```python
from build123d import *

# Parameters (mm, degrees)
F0_W     = 208
F0_H     = 115
F0_W_2   = 197.84
F0_H_2   = 109.92
F1_DEPTH = 4
F2_R     = 6
F3_SIZE  = 12.7
F4_W     = 15
F4_H     = 4
F5_DEPTH = 6
F6_W     = 15
F6_H     = 4
F7_DEPTH = 6
F8_R     = 3


with BuildPart() as f1:
    # F0 (on Top) → F1 (new body)
    with BuildSketch(Plane.XY):
        with Locations((104, 57.5)):
            Rectangle(F0_W, F0_H)
        with Locations((104, 57.5)):
            Rectangle(F0_W_2, F0_H_2, mode=Mode.SUBTRACT)
    extrude(amount=F1_DEPTH)

    # F2
    f2_edges = [f1.edges().sort_by_distance(p)[0] for p in [
        (0, 115, 2),
        (208, 115, 2),
        (208, 0, 2),
        (0, 0, 2),
    ]]
    fillet(f2_edges, radius=F2_R)

    # F3
    f3_edges = [f1.edges().sort_by_distance(p)[0] for p in [
        (5.08, 112.46, 2),
        (202.92, 2.54, 2),
        (202.92, 112.46, 2),
        (5.08, 2.54, 2),
    ]]
    chamfer(f3_edges, length=F3_SIZE)

    # F4 (on face) → F5 (join)
    with BuildSketch(Plane(origin=(0, 2.54, 0), x_dir=(-1, 0, 0), z_dir=(0, 1, 0))):
        with Locations((-104, 2)):
            Rectangle(F4_W, F4_H)
    extrude(amount=F5_DEPTH)

    # F6 (on face) → F7 (join)
    with BuildSketch(Plane.XZ.offset(-112.46)):
        with Locations((104, 2)):
            Rectangle(F6_W, F6_H)
    extrude(amount=F7_DEPTH)

    # F8
    f8_edges = [f1.edges().sort_by_distance(p)[0] for p in [
        (96.5, 106.46, 2),
        (111.5, 106.46, 2),
        (111.5, 8.54, 2),
        (96.5, 8.54, 2),
    ]]
    fillet(f8_edges, radius=F8_R)


solid = f1.part
```
For this review, take the finished solid that the model builds, in its own axes (mm). A direction names the side the tool comes from. Round coordinates to 2 decimals unless told otherwise and drop trailing zeros. Order: outer loops, then holes, each group sorted by start corner. A loop starts at its lowest first (then second) coordinate and runs counter-clockwise, first axis right, second up. Notation, with made-up numbers: (66.25, 70) -> (106.25, 70) arc R33 ccw to (106.25, 103) -> close; hole circle Ø7 at (44, 27.5). An arc over 180 degrees is marked (long way). Use a Markdown table: item, result.
Item 1: Draft analysis for pull direction Y (two halves, no side actions). For faces 1 (the flat face through (57, 2.54, 2)), 2 (the flat face through (104, 7, 4)), 3 (the cylindrical face through (1.711, 1.804, 2.028)), 4 (the cylindrical face through (1.711, 113.196, 2.028)), state which applies: +Y half, -Y half, draft (parallel to the pull), parting line (faces both ways), or undercut.
Resolved:
| item | result |
|---|---|
| face 1 | undercut |
| face 2 | draft |
| face 3 | -Y half |
| face 4 | +Y half |
Item 2: Take a section at B-B (x = 139.5). State the section outline as (y, z) points, plus the area to 3 significant figures.
Resolved:
| item | result |
|---|---|
| outline | (0, 0) -> (2.54, 0) -> (2.54, 4) -> (0, 4) -> close; (112.46, 0) -> (115, 0) -> (115, 4) -> (112.46, 4) -> close |
| area | 20.3 mm² |
Item 3: Machinability: for faces 5 (the flat face through (150, 2.54, 2)), 6 (the cylindrical face through (206.196, 113.289, 2.028)), which of the approach directions +Z, -Z, +X, -X, +Y, -Y give a long, thin tool a straight path to every point of the face, cutting with its end or side? Answer none if there is none.
Resolved:
| item | result |
|---|---|
| face 5 | +Z, -Z |
| face 6 | +Z, -Z, +X, +Y |
Item 4: Take a section at C-C (y = 38). State the section outline as (x, z) points, plus the area to 3 significant figures.
Resolved:
| item | result |
|---|---|
| outline | (0, 0) -> (5.08, 0) -> (5.08, 4) -> (0, 4) -> close; (202.92, 0) -> (208, 0) -> (208, 4) -> (202.92, 4) -> close |
| area | 40.6 mm² |
Item 5: For line 1 along X through (y, z) = (31.5, 3.3); line 2 along Y through (x, z) = (116.5, 3.25); line 3 along Y through (x, z) = (105.5, 1.5), list the stretches that pass through material, from the lowest coordinate up. Write a range as [from, to].
Resolved:
| item | result |
|---|---|
| line 1 | x = [0, 5.08], [202.92, 208] |
| line 2 | y = [0, 2.54], [112.46, 115] |
| line 3 | y = [0, 8.54], [106.46, 115] |
Item 6: For pin 1 (1.5 mm diameter, centred on y = 110.5, z = 1.5, fed in from +X); pin 2 (1.5 mm diameter, centred on y = 3.5, z = 1.5, fed in from -X); pin 3 (0.9 mm diameter, centred on y = 4, z = 2, fed in from +X), all flat-tipped, find the tip position at first contact; note any pin that passes through.
Resolved:
| item | result |
|---|---|
| pin 1 | stops at x = 207.95 |
| pin 2 | stops at x = 0.26 |
| pin 3 | stops at x = 207.8 |
Item 7: Take a section at A-A (z = 0.7). State the section outline as (x, y) points.
Resolved:
| item | result |
|---|---|
| outline | (0, 6) arc R6 ccw to (6, 0) -> (202, 0) arc R6 ccw to (208, 6) -> (208, 109) arc R6 ccw to (202, 115) -> (6, 115) arc R6 ccw to (0, 109) -> close; hole (5.08, 15.24) -> (17.78, 2.54) -> (96.5, 2.54) -> (96.5, 5.54) arc R3 cw to (99.5, 8.54) -> (108.5, 8.54) arc R3 cw to (111.5, 5.54) -> (111.5, 2.54) -> (190.22, 2.54) -> (202.92, 15.24) -> (202.92, 99.76) -> (190.22, 112.46) -> (111.5, 112.46) -> (111.5, 109.46) arc R3 cw to (108.5, 106.46) -> (99.5, 106.46) arc R3 cw to (96.5, 109.46) -> (96.5, 112.46) -> (17.78, 112.46) -> (5.08, 99.76) -> close |
